Input: part model. Units: mm. Frame: model coordinates. Coordinates: 2 decimals unless noted, no trailing zeros. Order: outer loops, then holes, each group sorted by start corner. A loop starts at its lowest first (then second) coordinate and runs counter-clockwise, first axis right, second up. Notation, with made-up numbers: (56, 80) - (78, 80) arc R27 cw to (78, 115) - close; hole circle Ø3 at (5, 31). An arc over 180 degrees is marked (long way). Answer as CSV lines item,"result". Start each with the question number.
Item 1: Section B-B (y = 1.15). Output: boundary loops of the cut face in (x, z), and give its area (3 significant figures).
Item 2: Section A-A (x = 8.5). Output: boundary loops of the cut face in (y, z).
Item 3: Material intervals for line 1 along X through (y, z) = (1.5, -8.5); line 2 along Z through (x, y) = (141.5, 1.75); line 3 along X through (y, z) = (1.55, -8), sorted ascending.
Item 4: First-contact query: pin 1 (2.5 mm diameter, centred on x = 141.5, z = -8.5, fed in from -Y). Flat tip, straight axial feed; report the tip coordinate or a pass-through.
Item 5: Draft query along X for faces 1 (the cylindrical face through (141.57, 1.27, -83.2)), 2 (the flat face through (74, 0, -46)). Return one class per face: +X half, -X half, draft (parallel to the pull), parting line (faces both ways), or undercut.
from build123d import *

# Parameters (mm, degrees)
SKETCH1_W           = 150
SKETCH1_H           = 90
BOSS_EXTRUDE1_DEPTH = 2.5
FILLET1_R           = 10
FILLET2_R           = 10
SKETCH2_R           = 1.7
CUT_EXTRUDE1_DEPTH  = 2.5


with BuildPart() as part:
    # Sketch1 → Boss-Extrude1 (new body)
    with BuildSketch(Plane(origin=(0, 0, 0), x_dir=(1, 0, 0), z_dir=(0, 1, 0))):
        with Locations((75, 45)):
            Rectangle(SKETCH1_W, SKETCH1_H)
    extrude(amount=BOSS_EXTRUDE1_DEPTH)

    # Fillet1
    # the kernel refuses this fillet: 10 mm, written as the material it takes off along each edge
    with BuildSketch(Plane(origin=(-16.535945694, 2.5, 0), x_dir=(0, -1, 0), z_dir=(1, 0, 0))) as fillet1_piece_1:
        with BuildLine():
            CenterArc((10, 6.614378278), FILLET1_R, 180, 41.409622109)
            Line((0, 6.614378278), (-0.2, 6.614378278))
            Line((-0.2, 6.614378278), (-0.2, 0))
            Line((-0.2, 0), (0, -0.2))
            ThreePointArc((0, -0.2), (1.25, -0.2), (2.35, -0.132287566))
            Line((2.35, -0.132287566), (2.5, 0))
        make_face()
    extrude(amount=183.071891388, mode=Mode.SUBTRACT)

    # Fillet2
    # the kernel refuses this fillet: 10 mm, written as the material it takes off along each edge
    with BuildSketch(Plane(origin=(166.535945694, 2.5, -90), x_dir=(0, -1, 0), z_dir=(-1, 0, 0))) as fillet2_piece_1:
        with BuildLine():
            CenterArc((10, 6.614378278), FILLET2_R, 180, 41.409622109)
            Line((0, 6.614378278), (-0.2, 6.614378278))
            Line((-0.2, 6.614378278), (-0.2, 0))
            Line((-0.2, 0), (0, -0.2))
            ThreePointArc((0, -0.2), (1.25, -0.2), (2.35, -0.132287566))
            Line((2.35, -0.132287566), (2.5, 0))
        make_face()
    extrude(amount=183.071891388, mode=Mode.SUBTRACT)

    # Sketch2 → Cut-Extrude1 (cut)
    with BuildSketch(Plane(origin=(0, 2.5, 0), x_dir=(1, 0, 0), z_dir=(0, 1, 0))):
        with Locations(Location((8.5, 81.5, 0), (0, 0, 270))):
            Circle(SKETCH2_R)
        with Locations(Location((8.5, 8.5, 0), (0, 0, 270))):
            Circle(SKETCH2_R)
        with Locations(Location((141.5, 81.5, 0), (0, 0, 270))):
            Circle(SKETCH2_R)
        with Locations(Location((141.5, 8.5, 0), (0, 0, 270))):
            Circle(SKETCH2_R)
    extrude(amount=-CUT_EXTRUDE1_DEPTH, mode=Mode.SUBTRACT)


solid = part.part
Determined:
1,outline,"(0, -88.4) - (150, -88.4) - (150, -1.6) - (0, -1.6) - close; hole circle Ø3.4 at (8.5, -81.5); hole circle Ø3.4 at (8.5, -8.5); hole circle Ø3.4 at (141.5, -81.5); hole circle Ø3.4 at (141.5, -8.5)"
1,area,"13,000 mm^2"
2,outline,"(0, -90) arc R10 ccw to (2.5, -83.39) - (2.5, -83.2) - (0, -83.2) - close; (0, -79.8) - (2.5, -79.8) - (2.5, -10.2) - (0, -10.2) - close; (0, -6.8) - (2.5, -6.8) - (2.5, -6.61) arc R10 ccw to (0, 0) - close"
3,line 1,"x = 0 to 6.8, 10.2 to 139.8, 143.2 to 150"
3,line 2,"z = -87.19 to -83.2, -79.8 to -10.2, -6.8 to -2.81"
3,line 3,"x = 0 to 6.88, 10.12 to 139.88, 143.12 to 150"
4,pin 1,"passes through"
5,face 1,"undercut"
5,face 2,"draft"
